Model file for the job. Use its own axes, mm. Coordinates: 2 decimals unless noted, no trailing zeros. Loops run counter-clockwise (first coordinate to the right, second up) from the corner with the lowest first, then second, coordinate; pieces in that order, holes last. Notation, with made-up numbers: M 55,54 L 63,54 A14 ccw 63,67 Z; hole C 48,-28 d6. An arc over 180 degrees is marked long. One line per question, with ' | ' between items. Start each with the question number.
```python
from build123d import *

# Parameters (mm, degrees)
F1_DEPTH = 3.175
F3_D     = 5
F5_D     = 3.3
F5_DEPTH = 6
F5_TIP   = 0.9914200214


with BuildPart() as f1:
    # F0 (on Right) → F1 (new body, symmetric)
    with BuildSketch(Plane.YZ):
        with BuildLine():
            Line((5, -0.0944561325), (4.9991077243, -0.0944561325))
            ThreePointArc((4.9991077243, -0.0944561325), (0, 5), (-4.9991077243, -0.0944561325))
            Line((-4.9991077243, -0.0944561325), (-5, -0.0944561325))
            Line((-5, -0.0944561325), (-5, -7.7014281414))
            Line((-5, -7.7014281414), (5, -7.7014281414))
            Line((5, -7.7014281414), (5, -0.0944561325))
        make_face()
    extrude(amount=F1_DEPTH, both=True)

    # F3 (through all)
    with Locations(Plane.YZ.offset(3.175)):
        with Locations((0, 0)):
            Hole(F3_D / 2)

    # F5
    with Locations(Plane(origin=(0, 0, -7.7014281414), x_dir=(1, 0, 0), z_dir=(0, 0, -1))):
        with Locations((0, 0)):
            Hole(F5_D / 2, depth=F5_DEPTH)
            with Locations((0, 0, -(F5_DEPTH + F5_TIP / 2))):  # 118° drill point
                Cone(0, F5_D / 2, F5_TIP, mode=Mode.SUBTRACT)


solid = f1.part
```
(1) Two-plate mould, pull along X, no slides. Class faces 1 (the face through (0, -5, -4)), 2 (the face through (3.175, 0, -3)), 3 (the face through (-1.524, 0.632, -4.749)), 4 (the face through (-3.175, 0, -3)): pulls with the +X half, pulls with the -X half, needs draft (parallel to the pull), parting line crosses it, or undercut.
(2) Band-saw the part on A-A on y = 0. Write the cut outline in (x, z) (3 decimals).
(3) Drill centre lines: line 1 (Y direction, x = 0, z = -5.2); line 2 (Y direction, x = 2.75, z = -2); line 3 (Z direction, x = 2.75, y = -0.5). Where is each one in solid material? Low to high. Write a range as [from, to].
(4) Band-saw the part on B-B on z = -1.5. Write the cut outline in (x, y) (3 decimals), then the cut area to 3 significant figures.
(5) Band-saw the part on C-C on z = -6.5. Write the cut outline in (x, y) (3 decimals).
Computed values:
1) face 1: needs draft | face 2: pulls with the +X half | face 3: undercut | face 4: pulls with the -X half
2) outline: M -3.175,-7.701 L -1.65,-7.701 L -1.65,-2.5 L -3.175,-2.5 Z; M -3.175,2.5 L 3.175,2.5 L 3.175,5 L -3.175,5 Z; M 1.65,-7.701 L 3.175,-7.701 L 3.175,-2.5 L 1.65,-2.5 Z
3) line 1: [-5, -1.65], [1.65, 5] | line 2: [-5, -1.5], [1.5, 5] | line 3: [-7.7, -2.45], [2.45, 4.97]
4) outline: M -3.175,-5 L 3.175,-5 L 3.175,-2 L -3.175,-2 Z; M -3.175,2 L 3.175,2 L 3.175,5 L -3.175,5 Z | area: 38.1 mm^2
5) outline: M -3.175,-5 L 3.175,-5 L 3.175,5 L -3.175,5 Z; hole C 0,0 d3.3
